from build123d import *

# Parameters (mm, degrees)
SKETCH1_R           = 1.25
BOSS_EXTRUDE1_DEPTH = 1
SKETCH2_W           = 25.7
SKETCH2_H           = 14.4
BOSS_EXTRUDE2_DEPTH = 1.5
SKETCH4_W           = 21.744
SKETCH4_H           = 11.204
BOSS_EXTRUDE3_DEPTH = 0.22


with BuildPart() as part:
    # Sketch1 → Boss-Extrude1 (new body)
    with BuildSketch(Plane(origin=(0, 0, 0), x_dir=(1, 0, 0), z_dir=(0, 1, 0))):
        with BuildLine():
            Line((-10.35, -13.65), (10.35, -13.65))
            ThreePointArc((10.35, -13.65), (12.683452378, -12.683452378), (13.65, -10.35))
            Line((13.65, -10.35), (13.65, 10.35))
            ThreePointArc((13.65, 10.35), (12.683452378, 12.683452378), (10.35, 13.65))
            Line((10.35, 13.65), (-10.35, 13.65))
            ThreePointArc((-10.35, 13.65), (-12.683452378, 12.683452378), (-13.65, 10.35))
            Line((-13.65, 10.35), (-13.65, -10.35))
            ThreePointArc((-13.65, -10.35), (-12.683452378, -12.683452378), (-10.35, -13.65))
        make_face()
        with Locations(Location((-10.35, 11.6, 0), (0, 0, 270))):
            Circle(SKETCH1_R, mode=Mode.SUBTRACT)
        with Locations(Location((10.35, 11.6, 0), (0, 0, 270))):
            Circle(SKETCH1_R, mode=Mode.SUBTRACT)
        with Locations(Location((10.35, -11.6, 0), (0, 0, 270))):
            Circle(SKETCH1_R, mode=Mode.SUBTRACT)
        with Locations(Location((-10.35, -11.6, 0), (0, 0, 270))):
            Circle(SKETCH1_R, mode=Mode.SUBTRACT)
    extrude(amount=BOSS_EXTRUDE1_DEPTH)

    # Sketch2 → Boss-Extrude2 (add)
    with BuildSketch(Plane(origin=(0, 1, 0), x_dir=(1, 0, 0), z_dir=(0, 1, 0))):
        with Locations((0, 2.43)):
            Rectangle(SKETCH2_W, SKETCH2_H)
    extrude(amount=BOSS_EXTRUDE2_DEPTH)

    # Sketch4 → Boss-Extrude3 (add)
    with BuildSketch(Plane(origin=(0, 2.5, 0), x_dir=(1, 0, 0), z_dir=(0, 1, 0))):
        with Locations((0, 2.43)):
            Rectangle(SKETCH4_W, SKETCH4_H)
    extrude(amount=BOSS_EXTRUDE3_DEPTH)


solid = part.part
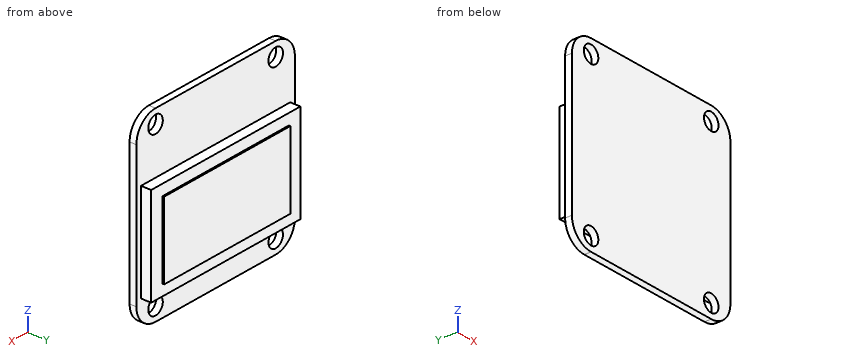
Source: CAD feature listing. Evaluate the final solid. Frame: model axes, mm. Coordinates: 2 decimals unless noted, no trailing zeros. Loops run counter-clockwise (first coordinate to the right, second up) from the corner with the lowest first, then second, coordinate; pieces in that order, holes last. Notation, with made-up numbers: (-18.75, 51.25) - (-10.75, 51.25) arc R12 ccw to (-10.75, 55.25) - close; hole circle Ø3 at (62.5, -37.75). An arc over 180 degrees is marked (long way). One line per item, written item: value. Start each with the question number.
1. Section A-A (z = -2.75). Return the cut outline in (x, y), and give its area (3 significant figures).
2. Section B-B (x = -9.75). Return the cut outline in (y, z).
3. Ray query, L1, parallel to X at y = 0.45, z = 11.6; L2, parallel to Z at x = -10, y = 0.35; L3, parallel to Y at x = -3, z = 12.5. Return the intervals inside material, ascending.
4. Section C-C (x = -7). Return the cut outline in (y, z).
5. Section D-D (z = -11.25). Return the cut outline in (x, y).
6. Contact query for a flat-ended pin moving along its axis: P1, Ø3, axis at x = -10.35, z = 11.6, coming from the +Y side. Output: stop coordinate, or through.
Verdict:
1. outline: (-13.65, 0) - (13.65, 0) - (13.65, 1) - (12.85, 1) - (12.85, 2.5) - (10.87, 2.5) - (10.87, 2.72) - (-10.87, 2.72) - (-10.87, 2.5) - (-12.85, 2.5) - (-12.85, 1) - (-13.65, 1) - close
1. area: 70.6 mm2
2. outline: (0, -13.65) - (1, -13.65) - (1, -12.7) - (0, -12.7) - close; (0, -10.5) - (1, -10.5) - (1, -9.63) - (2.5, -9.63) - (2.5, -8.03) - (2.72, -8.03) - (2.72, 3.17) - (2.5, 3.17) - (2.5, 4.77) - (1, 4.77) - (1, 10.5) - (0, 10.5) - close; (0, 12.7) - (1, 12.7) - (1, 13.65) - (0, 13.65) - close
3. L1: x = -13.4 to -11.6, -9.1 to 9.1, 11.6 to 13.4
3. L2: z = -13.65 to -12.8, -10.4 to 10.4, 12.8 to 13.65
3. L3: y = 0 to 1
4. outline: (0, -13.65) - (1, -13.65) - (1, -9.63) - (2.5, -9.63) - (2.5, -8.03) - (2.72, -8.03) - (2.72, 3.17) - (2.5, 3.17) - (2.5, 4.77) - (1, 4.77) - (1, 13.65) - (0, 13.65) - close
5. outline: (-13.52, 0) - (-11.55, 0) - (-11.55, 1) - (-13.52, 1) - close; (-9.15, 0) - (9.15, 0) - (9.15, 1) - (-9.15, 1) - close; (11.55, 0) - (13.52, 0) - (13.52, 1) - (11.55, 1) - close
6. P1: stops at y = 1
